Autodesk Inventor part; units mm, degrees
ref_plane "YZ Plane" through (0, 0, 0) normal (1, 0, 0) x (0, 1, 0)
ref_plane "XZ Plane" through (0, 0, 0) normal (0, 1, 0) x (-1, 0, 0)
ref_plane "XY Plane" through (0, 0, 0) normal (0, 0, 1) x (1, 0, 0)
sketch "Boceto1" plane through (0, 0, 0) normal (0, 0, 1) x (1, 0, 0)
  line L0 (0, 0) -> (50, 0)
  line L1 (50, 0) -> (50, 26)
  line L2 (50, 26) -> (26, 26)
  line L3 (0, 26) -> (0, 0)
  line L4 (0, 0) -> (26, 0)
  line L5 (26, 26) -> (26, 50)
  line L6 (26, 50) -> (0, 50)
  line L7 (0, 50) -> (0, 0)
  line L8 (0, 0) -> (50, 0)
  line L9 (50, 0) -> (50, 3)
  line L10 (50, 3) -> (0, 3)
  line L11 (0, 3) -> (0, 0)
  line L12 (0, 50) -> (3, 50)
  line L13 (3, 50) -> (3, 0)
  line L14 (3, 0) -> (0, 0)
  line L15 (0, 0) -> (0, 50)
  line L16 (26, 50) -> (23, 50)
  line L17 (23, 50) -> (23, 24)
  line L18 (23, 24) -> (26, 24)
  line L19 (26, 24) -> (26, 50)
  line L20 (50, 26) -> (23, 26)
  line L21 (23, 26) -> (23, 23)
  line L22 (23, 23) -> (50, 23)
  line L23 (50, 23) -> (50, 26)
  line L24 (23, 50) -> (1.5, 50)
  line L25 (3, 3) -> (50, 3)
  line L26 (50, 23) -> (23, 23)
  point P0 (3, 3)
  dimension "d0" = 50
  dimension "d1" = 26
  dimension "d2" = 26
  dimension "d3" = 50
  dimension "d4" = 50
  dimension "d5" = 3
  dimension "d6" = 3
  dimension "d7" = 50
  dimension "d8" = 3
  dimension "d9" = 26
  dimension "d10" = 27
  dimension "d11" = 3
extrude "Extrusión1" add sketch "Boceto1" along normal blind 26 contours L3 L10 L13 L0 | L13 L10 L1 L0
extrude "Extrusión2" add sketch "Boceto1" along normal blind 26 contours L3 L7 L6 L13 L10
extrude "Extrusión3" add sketch "Boceto1" along normal blind 26 contours L22 L21 L18 L19 L2 L1 | L20 L19 L18 L17
extrude "Extrusión4" add sketch "Boceto1" along normal blind 26 contours L6 L5 L20 L17
sketch "Boceto2" plane through (0, 0, 26) normal (0, 0, 1) x (1, 0, 0)
  line L0 (3, 50) -> (0, 50)
  line L1 (26, 50) -> (23, 50)
  line L2 (0, 50) -> (26, 50)
  line L3 (3, 50) -> (23, 50)
  line L4 (23, 50) -> (23, 23)
  line L5 (23, 23) -> (50, 23)
  line L6 (23, 23) -> (50, 23)
  line L7 (50, 0) -> (50, 3)
  line L8 (50, 23) -> (50, 3)
  line L9 (50, 3) -> (3, 3)
  line L10 (50, 3) -> (3, 3)
  line L11 (3, 3) -> (3, 50)
  point P0 (0, 0)
extrude "Extrusión5" add sketch "Boceto2" against normal blind 3
extrude "Extrusión6" add sketch "Boceto1" along normal blind 3 contours L13 L6 L17 L21 L22 L1 L10
sketch "Boceto3" plane through (0, 0, 26) normal (0, 0, 1) x (1, 0, 0)
  line L0 (0, 0) -> (50, 0)
  line L1 (0, 0) -> (26, 0)
  line L2 (0, 0) -> (26, 0) construction
  line L3 (50, 26) -> (26, 26)
  line L4 (26, 0) -> (26, 26)
  line L5 (26, 26) -> (0, 26)
  line L6 (3, 3) -> (3, 50)
  line L7 (0, 26) -> (0, 0)
  line L8 (3, 3) -> (50, 3)
  line L9 (3, 3) -> (23, 3)
  line L10 (23, 3) -> (23, 23)
  line L11 (23, 23) -> (3, 23)
  line L12 (3, 23) -> (3, 3)
  dimension "d24" = 26
  dimension "d25" = 0
  dimension "d26" = 20
  dimension "d27" = 20
extrude "Extrusión7" cut sketch "Boceto3" against normal blind 3 contours L8 L6 L11 L10
sketch "Boceto4" plane through (0, 0, 26) normal (0, 0, 1) x (1, 0, 0)
  line L0 (0, 0) -> (26, 0)
  line L1 (0, 0) -> (50, 0)
  line L2 (0, 0) -> (26, 0) construction
  line L3 (26, 0) -> (26, 26)
  line L4 (26, 26) -> (0, 26)
  line L5 (3, 23) -> (23, 23)
  line L6 (0, 50) -> (0, 0)
  line L7 (0, 26) -> (0, 0)
  line L8 (50, 23) -> (23, 23)
  line L9 (3, 23) -> (23, 23)
  line L10 (23, 23) -> (23, 3)
  line L11 (23, 23) -> (23, 3)
  line L12 (50, 3) -> (3, 3)
  line L13 (23, 3) -> (3, 3)
  line L14 (3, 3) -> (3, 23)
  dimension "d30" = 26
  dimension "d31" = 0
  dimension "d32" = 26
  dimension "d33" = 90
extrude "Extrusión8" add sketch "Boceto4" along normal blind 35 contours L6 L4 L3 L8 L5 L14 L12 L0 | L12 L10 L8 L3
sketch "Boceto5" plane through (26, 0, 26) normal (1, 0, 0) x (0, 0, -1)
  circle A0 centre (-23.5, 13) radius 1.75
  circle A1 centre (-11.5, 13) radius 1.75
  line L0 (0, 26) -> (-35, 26)
  line L1 (-35, 0) -> (-35, 26)
  line L2 (0, 0) -> (0, 26)
  point P0 (26, 0)
  dimension "d36" = 3.5
  dimension "d37" = 3.5
  dimension "d38" = 13
  dimension "d39" = 13
  dimension "d40" = 12
  dimension "d41" = 11.5
  dimension "d42" = 35
  dimension "d43" = 11.5
sketch "Boceto6" plane through (50, 0, 26) normal (1, 0, 0) x (0, 0, -1)
  line L0 (26, 26) -> (0, 26)
  line L1 (26, 26) -> (26, 50)
  line L2 (0, 26) -> (26, 26)
  line L3 (26, 50) -> (26, 0)
  line L4 (26, 26) -> (26, 0)
  line L5 (26, 0) -> (0, 0)
  line L6 (26, 0) -> (-35, 0)
  line L7 (23, 23) -> (3, 23)
  line L8 (3, 23) -> (23, 23)
  line L9 (23, 23) -> (23, 3)
  line L10 (23, 3) -> (3, 3)
  line L11 (23, 3) -> (-35, 3)
  line L12 (-35, 23) -> (3, 23)
  line L13 (3, 3) -> (3, 23)
  line L14 (0, 26) -> (0, 0)
extrude "Extrusión9" add sketch "Boceto6" along normal blind 11 contours L3 L5 L14 L11 L10 L9 L7 L12 L0 | L12 L13 L11 L14
sketch "Boceto7" plane through (0, 50, 26) normal (0, 1, 0) x (1, 0, 0)
  line L0 (3, 3) -> (23, 3)
  line L1 (3, 3) -> (23, 3)
  line L2 (23, 3) -> (23, 23)
  line L3 (23, 23) -> (3, 23)
  line L4 (3, 23) -> (3, 3)
  line L5 (26, 26) -> (26, 0)
  line L6 (26, 26) -> (0, 26)
  line L7 (0, 26) -> (0, 0)
  line L8 (0, 0) -> (26, 0)
  line L9 (26, 0) -> (26, 26)
  dimension "d46" = 20
  dimension "d47" = 20
  dimension "d48" = 26
  dimension "d49" = 26
extrude "Extrusión10" add sketch "Boceto7" along normal blind 11
sketch "Boceto8" plane through (0, 0, 26) normal (0, 0, 1) x (1, 0, 0)
  circle A0 centre (49.5, 13) radius 1.75
  circle A1 centre (37.5, 13) radius 1.75
  line L0 (61, 26) -> (61, 0)
  line L1 (26, 26) -> (61, 26)
  point P0 (0, 0)
  dimension "d52" = 3.5
  dimension "d53" = 3.5
  dimension "d54" = 11.5
  dimension "d55" = 12
  dimension "d56" = 13
  dimension "d57" = 13
extrude "Extrusión11" cut sketch "Boceto5" against normal up to next contours A0
extrude "Extrusión12" cut sketch "Boceto5" against normal up to next contours A1
extrude "Extrusión13" cut sketch "Boceto8" against normal up to next contours A1
extrude "Extrusión14" cut sketch "Boceto8" against normal up to next contours A0
sketch "Boceto9" plane through (0, 0, 26) normal (0, 0, 1) x (1, 0, 0)
  circle A0 centre (13, 37.5) radius 1.75
  circle A1 centre (13, 49.5) radius 1.75
  line L0 (0, 26) -> (0, 61)
  line L1 (0, 61) -> (26, 61)
  point P0 (0, 0)
  dimension "d66" = 3.5
  dimension "d67" = 3.5
  dimension "d68" = 13
  dimension "d69" = 13
  dimension "d70" = 11.5
  dimension "d71" = 12
sketch "Boceto10" plane through (26, 26, 26) normal (1, 0, 0) x (0, 0, -1)
  circle A0 centre (13, 23.5) radius 1.75
  circle A1 centre (13, 11.5) radius 1.75
  line L0 (0, 0) -> (0, 35)
  line L1 (0, 35) -> (26, 35)
  point P0 (26, -26)
  dimension "d72" = 3.5
  dimension "d73" = 3.5
  dimension "d74" = 13
  dimension "d75" = 13
  dimension "d76" = 12
  dimension "d77" = 11.5
extrude "Extrusión15" cut sketch "Boceto9" against normal up to next contours A1
extrude "Extrusión16" cut sketch "Boceto9" against normal up to next contours A0
extrude "Extrusión17" cut sketch "Boceto10" against normal up to next contours A0
extrude "Extrusión18" cut sketch "Boceto10" against normal up to next contours A1
sketch "Boceto12" plane through (3, 3, 61) normal (0, 1, 0) x (1, 0, 0)
  line L0 (58, 58) -> (0, 58)
  line L1 (0, 58) -> (0, 0)
  line L2 (20, 0) -> (0, 0)
  line L3 (20, 0) -> (20, 38)
  line L4 (20, 38) -> (58, 38)
  line L5 (58, 58) -> (58, 38)
  line L6 (23, 35) -> (23, 61)
  line L7 (23, 61) -> (-3, 61)
  line L8 (-3, 61) -> (-3, 35)
  line L9 (-3, 35) -> (23, 35)
  line L10 (0, 38) -> (0, 58)
  line L11 (0, 58) -> (20, 58)
  line L12 (20, 58) -> (20, 38)
  line L13 (20, 38) -> (0, 38)
  line L14 (23, 35) -> (23, 61)
  line L15 (23, 61) -> (-3, 61)
  line L16 (-3, 61) -> (-3, 35)
  line L17 (-3, 35) -> (23, 35)
  line L18 (0, 38) -> (0, 58)
  line L19 (0, 58) -> (20, 58)
  line L20 (20, 58) -> (20, 38)
  line L21 (20, 38) -> (0, 38)
  line L22 (20, 58) -> (20, 38)
  line L23 (0, 38) -> (0, 58)
  line L24 (20, 38) -> (0, 38)
  line L25 (0, 0) -> (20, 0)
  line L26 (0, 58) -> (20, 58)
  line L27 (58, 58) -> (0, 58)
  line L28 (20, 58) -> (58, 58)
  line L29 (58, 38) -> (58, 58)
properties part number "esquina20mm"
The model under review builds one solid part; all positions refer to its coordinate system, in mm. A direction names the side the tool comes from. Give positions to 0.01 mm unless a question says otherwise; leave off trailing zeros. Write each loop counter-clockwise with the first axis right and the second up, starting at its lowest first coordinate (ties: lowest second). Pieces come first, ordered by that corner, then holes. Notation, with made-up numbers: (80.25, 87) -> (86.25, 87) arc R31 cw to (86.25, 117) -> close; hole circle Ø4 at (35.5, 4). An arc over 180 degrees is marked (long way). Answer in a Markdown table with one row per item.
1) For L1, parallel to Y at x = 25.15, z = 13; L2, parallel to Y at x = 42, z = 11; L3, parallel to Y at x = 37.5, z = 25.2, list the stretches that pass through material, from the lowest coordinate up. Write a range as [from, to].
Worked answers:
| item | result |
|---|---|
| L1 | [0, 3], [23, 35.75], [39.25, 47.75], [51.25, 61] |
| L2 | [0, 3], [23, 26] |
| L3 | [0, 11.25], [14.75, 26] |
2) Add section A-A on x = 41. State the section outline as (y, z) points, plus the area to 3 significant figures.
Worked answers:
| item | result |
|---|---|
| outline | (0, 0) -> (26, 0) -> (26, 26) -> (0, 26) -> close; hole (3, 3) -> (23, 3) -> (23, 23) -> (3, 23) -> close |
| area | 276 mm² |
3) Add section B-B on y = 13. State the section outline as (x, z) points.
Worked answers:
| item | result |
|---|---|
| outline | (0, 0) -> (61, 0) -> (61, 3) -> (3, 3) -> (3, 61) -> (0, 61) -> close; (23, 23) -> (35.75, 23) -> (35.75, 26) -> (26, 26) -> (26, 35.75) -> (23, 35.75) -> close; (23, 39.25) -> (26, 39.25) -> (26, 47.75) -> (23, 47.75) -> close; (23, 51.25) -> (26, 51.25) -> (26, 61) -> (23, 61) -> close; (39.25, 23) -> (47.75, 23) -> (47.75, 26) -> (39.25, 26) -> close; (51.25, 23) -> (61, 23) -> (61, 26) -> (51.25, 26) -> close |
4) Mouldability with a two-part tool opening along X and no side actions: class faces 5 (the flat face through (23, 42, 13)), 6 (the flat face through (24, 23, 0)), 7 (the flat face through (26, 43, 13)) as +X half, -X half, draft (parallel to the pull), parting line (faces both ways), or undercut.
Worked answers:
| item | result |
|---|---|
| face 5 | undercut |
| face 6 | draft |
| face 7 | +X half |
5) Clearance check with flat-ended pins moving along their axes: P1, Ø8, axis at x = 45.5, y = 14, coming from the +Z side; P2, Ø2, axis at x = 13, y = 49.5, coming from the +Z side; P3, Ø8, axis at y = 14.5, z = 36.5, coming from the +X side. State where each tip first meets the part, or that it passes through.
Worked answers:
| item | result |
|---|---|
| P1 | z = 26 |
| P2 | z = 3 |
| P3 | x = 26 |
6) Tool access review of faces 1 (the flat face through (42, 23, 13)), 2 (the flat face through (44, 26, 13)), 3 (the cylindrical face through (38.4, 14.5, 24.5)), 4 (the flat face through (13, 26, 43)): name each direction out of +Z, -Z, +X, -X, +Y, -Y from which nothing blocks a thin tool from reaching the whole face with its end or side.
Worked answers:
| item | result |
|---|---|
| face 1 | +X |
| face 2 | +Z, -Z, +X, +Y |
| face 3 | +Z |
| face 4 | +Z, +X, -X, +Y |
7) Add section D-D on x = 19.5. State the section outline as (y, z) points, plus the area to 3 significant figures.
Worked answers:
| item | result |
|---|---|
| outline | (0, 0) -> (61, 0) -> (61, 3) -> (3, 3) -> (3, 61) -> (0, 61) -> close; (23, 23) -> (61, 23) -> (61, 26) -> (26, 26) -> (26, 61) -> (23, 61) -> close |
| area | 576 mm² |
